from build123d import *

# Parameters (mm, degrees)
SKETCH1_R           = 78.359
SKETCH1_R_2         = 76.2
BOSS_EXTRUDE1_DEPTH = 1219.2
SKETCH2_W           = 3.175
SKETCH2_H           = 292.1
CUT_EXTRUDE2_DEPTH  = 1225.225839362
CIRPATTERN1_COUNT   = 4


with BuildPart() as part:
    # Sketch1 → Boss-Extrude1 (new body)
    with BuildSketch(Plane(origin=(0, 0, 0), x_dir=(1, 0, 0), z_dir=(0, 1, 0))):
        with Locations(Location((0, 0, 0), (0, 0, 90))):
            Circle(SKETCH1_R)
        with Locations(Location((0, 0, 0), (0, 0, 90))):
            Circle(SKETCH1_R_2, mode=Mode.SUBTRACT)
    extrude(amount=BOSS_EXTRUDE1_DEPTH)

    # Sketch2 → Cut-Extrude2 (cut, through all)
    with BuildSketch(Plane.XY):
        with Locations((0, 146.05)):
            Rectangle(SKETCH2_W, SKETCH2_H)
    cut_extrude2 = extrude(amount=CUT_EXTRUDE2_DEPTH, mode=Mode.SUBTRACT)

    # CirPattern1: Cut-Extrude2 ×4 about axis
    cirpattern1_axis = Axis((0, 0, 0), (0, 1, 0))
    for i in range(1, CIRPATTERN1_COUNT):
        add(cut_extrude2.rotate(cirpattern1_axis, i * 360 / CIRPATTERN1_COUNT), mode=Mode.SUBTRACT)


solid = part.part
Input: part model. Units: mm. Frame: model coordinates. Round coordinates to 2 decimals unless told otherwise and drop trailing zeros. Write each loop counter-clockwise with the first axis right and the second up, starting at its lowest first coordinate (ties: lowest second). Pieces come first, ordered by that corner, then holes.
1) Draft query along X for faces 1 (the cylindrical face through (46.367, 601.066, 60.47)), 2 (the cylindrical face through (-23.54, 601.07, -74.74)), 3 (the flat face through (75, 1219.2, -17)). Return one class per face: pulls with the +X half, pulls with the -X half, needs draft (parallel to the pull), parting line crosses it, or undercut.
2) Ray query, L1, parallel to X at y = 387, z = 0; L2, parallel to Z at x = -63.5, y = 1078.5; L3, parallel to Z at x = -52, y = 892. Return the intervals inside material, ascending.
3) Cut plane C-C (y = 1121.5). Return the cut outline in (x, z).
4) Cut plane A-A (x = -42). Return the cut outline in (y, z).
5) Contact query for flat-ended pins moving along their axis: P1, Ø12, axis at y = 682, z = 54, coming from the +X side; P2, Ø0.7, axis at x = -0.5, z = -77, coming from the -Y side; P3, Ø2, axis at y = 254, z = -2, coming from the +X side. Output: stop coordinate, or through.
6) Cut plane B-B (z = 63.5). Return the cut outline in (x, y), then the cut area to 3 significant figures.
Geometry says:
1. face 1: undercut
1. face 2: parting line crosses it
1. face 3: needs draft
2. L1: x = -78.36 to -76.2, 76.2 to 78.36
2. L2: z = -45.91 to -42.12, 42.12 to 45.91
2. L3: z = -58.62 to -55.7, 55.7 to 58.62
3. outline: circle Ø156.72 at (0, 0); hole circle Ø152.4 at (0, 0)
4. outline: (0, -66.15) - (1219.2, -66.15) - (1219.2, -63.58) - (0, -63.58) - close; (0, 63.58) - (1219.2, 63.58) - (1219.2, 66.15) - (0, 66.15) - close
5. P1: stops at x = 61.94
5. P2: stops at y = 292.1
5. P3: stops at x = 78.34
6. outline: (-45.91, 0) - (-42.12, 0) - (-42.12, 1219.2) - (-45.91, 1219.2) - close; (42.12, 0) - (45.91, 0) - (45.91, 1219.2) - (42.12, 1219.2) - close
6. area: 9,240 mm2
